Geometry: final body of the model. Coordinates: model frame, mm. Face numbers are marked on the shaded views. A direction names the side the tool comes from. Round coordinates to 2 decimals unless told otherwise and drop trailing zeros. Write each loop counter-clockwise with the first axis right and the second up, starting at its lowest first coordinate (ties: lowest second). Pieces come first, ordered by that corner, then holes. Notation, with made-up numbers: M 60,80 L 69,80 A11 ccw 69,90 Z; hole C -18.75,-15.5 d9. An arc over 180 degrees is marked long. Put each result on its own line as item: value. Start each with the question number.
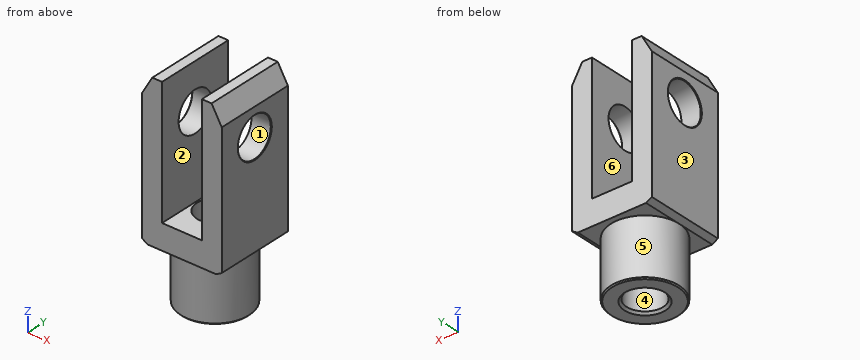
```python
from build123d import *
from OCP.BRepFilletAPI import BRepFilletAPI_MakeChamfer

# Parameters (mm, degrees)
SKETCH2_R           = 30
BOSS_EXTRUDE1_DEPTH = 50
SKETCH3_W           = 70
SKETCH3_H           = 70
BOSS_EXTRUDE2_DEPTH = 134
SKETCH4_W           = 35
SKETCH4_H           = 70
CUT_EXTRUDE1_DEPTH  = 112
SKETCH5_R           = 16
CUT_EXTRUDE2_DEPTH  = 72
CHAMFER1_SIZE       = 15.5
CHAMFER1_SIZE2      = 8.948929172
SKETCH6_R           = 17.5
CUT_EXTRUDE3_DEPTH  = 70
CHAMFER2_SIZE       = 0.5
CHAMFER4_SIZE       = 1
CHAMFER6_SIZE       = 2
CHAMFER7_SIZE       = 5
CHAMFER7_SIZE_2     = 2.886751346


with BuildPart() as part:
    # Sketch2 → Boss-Extrude1 (new body)
    with BuildSketch(Plane.XY):
        Circle(SKETCH2_R)
    extrude(amount=BOSS_EXTRUDE1_DEPTH)

    # Sketch3 → Boss-Extrude2 (add)
    with BuildSketch(Plane.XY.offset(50)):
        Rectangle(SKETCH3_W, SKETCH3_H)
    extrude(amount=BOSS_EXTRUDE2_DEPTH)

    # Sketch4 → Cut-Extrude1 (cut)
    with BuildSketch(Plane.XY.offset(184)):
        Rectangle(SKETCH4_W, SKETCH4_H)
    extrude(amount=-CUT_EXTRUDE1_DEPTH, mode=Mode.SUBTRACT)

    # Sketch5 → Cut-Extrude2 (cut)
    with BuildSketch(Plane(origin=(0, 0, 0), x_dir=(-1, 0, 0), z_dir=(0, 0, -1))):
        Circle(SKETCH5_R)
    extrude(amount=-CUT_EXTRUDE2_DEPTH, mode=Mode.SUBTRACT)

    # Chamfer1: one chamfer whose edges measure the first distance from different faces: ONE call of the kernel's chamfer builder (chamfer() names one face for all edges)
    chamfer1_edges_1 = [part.edges().sort_by_distance(p)[0] for p in [
        (-35, 0, 184),
    ]]
    chamfer1_side_1 = [part.faces().sort_by_distance(p)[0] for p in [
        (-35, 0, 117),
    ]]
    chamfer1_edges_2 = [part.edges().sort_by_distance(p)[0] for p in [
        (35, 0, 184),
    ]]
    chamfer1_side_2 = [part.faces().sort_by_distance(p)[0] for p in [
        (35, 0, 117),
    ]]
    chamfer1 = BRepFilletAPI_MakeChamfer(part.part.solid().wrapped)
    for e in chamfer1_edges_1:
        chamfer1.Add(CHAMFER1_SIZE, CHAMFER1_SIZE2, e.wrapped, chamfer1_side_1[0].wrapped)  # the first distance lies on this face
    for e in chamfer1_edges_2:
        chamfer1.Add(CHAMFER1_SIZE, CHAMFER1_SIZE2, e.wrapped, chamfer1_side_2[0].wrapped)  # the first distance lies on this face
    add(Compound.cast(chamfer1.Shape()), mode=Mode.REPLACE)

    # Sketch6 → Cut-Extrude3 (cut)
    with BuildSketch(Plane(origin=(35, 0, 0), x_dir=(0, 0, -1), z_dir=(1, 0, 0))):
        with Locations(Location((-144, 0, 0), (0, 0, 90))):
            Circle(SKETCH6_R)
    extrude(amount=-CUT_EXTRUDE3_DEPTH, mode=Mode.SUBTRACT)

    # Chamfer2
    chamfer2_edges = [part.edges().sort_by_distance(p)[0] for p in [
        (-35, -17.5, 144),
        (35, -17.5, 144),
    ]]
    chamfer(chamfer2_edges, length=CHAMFER2_SIZE)

    # Chamfer4
    chamfer4_edges = [part.edges().sort_by_distance(p)[0] for p in [
        (-30, 0, 0),
    ]]
    chamfer(chamfer4_edges, length=CHAMFER4_SIZE)

    # Chamfer6
    chamfer6_edges = [part.edges().sort_by_distance(p)[0] for p in [
        (16, 0, 0),
    ]]
    chamfer(chamfer6_edges, length=CHAMFER6_SIZE)

    # Chamfer7
    chamfer7_edges_1 = [part.edges().sort_by_distance(p)[0] for p in [
        (-35, 0, 50),
    ]]
    chamfer7_side_1 = [part.faces().sort_by_distance(p)[0] for p in [
        (-34.942264973, 0, 50),
    ]]
    chamfer7_edges_2 = [part.edges().sort_by_distance(p)[0] for p in [
        (35, 0, 50),
    ]]
    chamfer7_side_2 = [part.faces().sort_by_distance(p)[0] for p in [
        (34.942264973, 0, 50),
    ]]
    chamfer7 = BRepFilletAPI_MakeChamfer(part.part.solid().wrapped)
    for e in chamfer7_edges_1:
        chamfer7.Add(CHAMFER7_SIZE - 0.0001, CHAMFER7_SIZE_2 - 0.0001, e.wrapped, chamfer7_side_1[0].wrapped)
    for e in chamfer7_edges_2:
        chamfer7.Add(CHAMFER7_SIZE - 0.0001, CHAMFER7_SIZE_2 - 0.0001, e.wrapped, chamfer7_side_2[0].wrapped)
    add(Compound.cast(chamfer7.Shape()), mode=Mode.REPLACE)  # a hair under: the kernel refuses the full size


solid = part.part
```
1) Section B-B, the plane x = 0. Output: boundary loops of the cut face in (y, z).
2) Draft query along X for the marked faces 1, 2 and 3. Return one class per face: +X half, -X half, draft (parallel to the pull), parting line (faces both ways), or undercut.
3) Access query for the marked faces 4, 5 and 6. Directions: +Z, -Z, +X, -X, +Y, -Y. A direction counts if a zero-diameter tool reaches every point of the face in a straight line with its end or side. Return the directions, or none.
4) First-contact query: pin 1 (4 mm diameter, centred on x = 5.5, y = -27.5, fed in from +Z); pin 2 (5 mm diameter, centred on y = 25.5, z = 26, fed in from -X). Flat tips, straight axial feed; report the tip coordinate or a pass-through.
5) Section D-D, the plane y = 0. Give the number of separate pieces and of enclosed holes in the cut face, and give its area (3 significant figures).
6) Section C-C, the plane z = 93. Output: boundary loops of the cut face in (x, y), and give its area (3 significant figures).
7) Ray query, probe 1 along Z at (x, y) = (-22.25, 0); probe 2 along Y at (x, z) = (0, 17); probe 3 along X at (y, z) = (18, 90.5). Return the intervals inside material, ascending.
8) Section A-A, the plane z = 144. Output: boundary loops of the cut face in (x, y), and give its area (3 significant figures).
Solved:
1. outline: M -35,50 L -30,50 L -30,1 L -29,0 L -18,0 L -16,2 L -16,72 L -35,72 Z; M 16,2 L 18,0 L 29,0 L 30,1 L 30,50 L 35,50 L 35,72 L 16,72 Z
2. face 1: draft
2. face 2: undercut
2. face 3: -X half
3. face 4: +Z, -Z
3. face 5: -Z
3. face 6: +Z, +Y, -Y
4. pin 1: stops at z = 72
4. pin 2: stops at x = -19.26
5. separate pieces: 4
5. enclosed holes: 0
5. area: 4,770 mm2
6. outline: M -35,-35 L -17.5,-35 L -17.5,35 L -35,35 Z; M 17.5,-35 L 35,-35 L 35,35 L 17.5,35 Z
6. area: 2,450 mm2
7. probe 1: z = 0 to 126.5, 161.5 to 184
7. probe 2: y = -30 to -16, 16 to 30
7. probe 3: x = -35 to -17.5, 17.5 to 35
8. outline: M -35,-35 L -17.5,-35 L -17.5,-17.5 L -34.5,-17.5 L -35,-18 Z; M -35,18 L -34.5,17.5 L -17.5,17.5 L -17.5,35 L -35,35 Z; M 17.5,-35 L 35,-35 L 35,-18 L 34.5,-17.5 L 17.5,-17.5 Z; M 17.5,17.5 L 34.5,17.5 L 35,18 L 35,35 L 17.5,35 Z
8. area: 1,220 mm2
